Input: dimensioned drawing with shaded views. Units: mm. Origin: part minimum x, y, z. A direction names the side the tool comes from. Give positions to 0.01 mm unless a question says otherwise; leave off trailing zeros. Loops run counter-clockwise (first coordinate to the right, second up) from the corner with the lowest first, then second, coordinate; pieces in that order, holes last. Notation, with made-up numbers: M 31,-9.5 L 69,-9.5 A12 ccw 69,5.5 Z; hole C 39.25,32 d7. An arc over 180 degrees is marked long. Use CSV: the item, a comma, the result in double quotes. Start each with the question number.
Q1. Section B-B, the plane y = 9.25. Output: boundary loops of the cut face in (x, z), plus the area to 3 significant figures.
Q2. Reachability of the marked faces 4, 5, 6 and 7 from +Z, -Z, +X, -X, +Y, -Y: full face, straight path, thin tool, end or side. Return the list, or none.
Q3. Material intervals for line 1 along Z through (x, y) = (10.5, 17.5); line 2 along Y through (x, z) = (13.5, 5.5); line 3 along X through (y, z) = (3.75, 3), sorted ascending.
Q4. Section D-D, the plane x = 3.25. Output: boundary loops of the cut face in (y, z), plus the area to 3 significant figures.
Q5. Pull-direction query (Y, two-part tool) for the marked faces 1, 2 and 3; classes: released by +Y, released by -Y, zero draft, split by the parting line, or undercut.
Q6. Section A-A, the plane x = 12.5. Output: boundary loops of the cut face in (y, z).
Q7. Section C-C, the plane z = 5.5. Output: boundary loops of the cut face in (x, y).
Q8. Pin query (flat end, axial travel): pin 1 (0.8 mm diameter, centred on x = 26.5, y = 4.5, fed in from -Z); pin 2 (1.2 mm diameter, centred on x = 14, y = 1.5, fed in from -Z); pin 3 (1.5 mm diameter, centred on x = 22.5, z = 1.5, fed in from +Y); pin 4 (3 mm diameter, centred on x = 13, y = 1.5, fed in from +Z). Return the tip coordinate at first contact, or that it passes through.
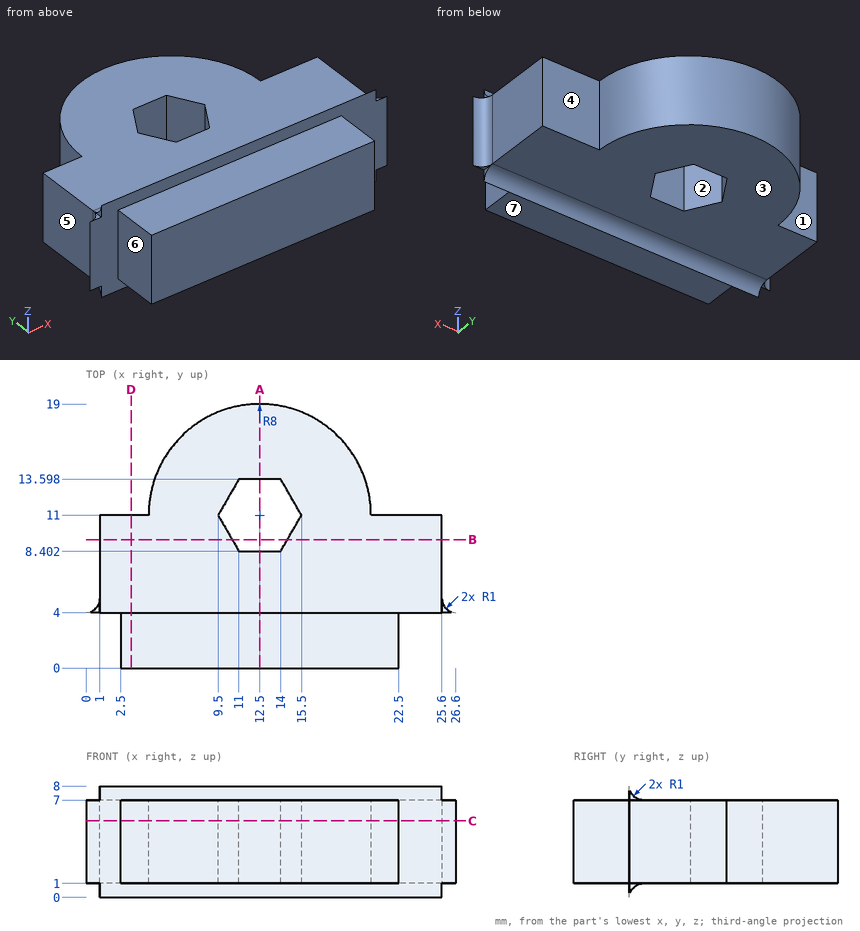
A:
1,outline,"M 1,1 L 10.51,1 L 10.51,7 L 1,7 Z; M 14.49,1 L 25.6,1 L 25.6,7 L 14.49,7 Z"
1,area,"124 mm^2"
2,face 4,"+Z, -Z, +X, +Y"
2,face 5,"+Z, -Z, -X, +Y"
2,face 6,"+Z, -Z, -X, -Y"
2,face 7,"-Z, +X, -X, -Y"
3,line 1,"1 to 7"
3,line 2,"0 to 8.4, 13.6 to 18.94"
3,line 3,"2.5 to 22.5"
4,outline,"M 0,1 L 4,1 L 4,0 A1 cw 5,1 L 11,1 L 11,7 L 5,7 A1 cw 4,8 L 4,7 L 0,7 Z"
4,area,"66.4 mm^2"
5,face 1,"released by +Y"
5,face 2,"undercut"
5,face 3,"zero draft"
6,outline,"M 0,1 L 4,1 L 4,0 A1 cw 5,1 L 8.4,1 L 8.4,7 L 5,7 A1 cw 4,8 L 4,7 L 0,7 Z; M 13.6,1 L 19,1 L 19,7 L 13.6,7 Z"
7,outline,"M 0,4 L 2.5,4 L 2.5,0 L 22.5,0 L 22.5,4 L 26.6,4 A1 cw 25.6,5 L 25.6,11 L 20.5,11 A8 ccw 4.5,11 L 1,11 L 1,5 A1 cw Z; hole M 9.5,11 L 11,8.4 L 14,8.4 L 15.5,11 L 14,13.6 L 11,13.6 Z"
8,pin 1,"through"
8,pin 2,"z = 1"
8,pin 3,"y = 11"
8,pin 4,"z = 7"
